from build123d import *

# Parameters (mm, degrees)
PAD_DEPTH       = 1.7
SKETCH002_W     = 6
SKETCH002_H     = 6
PAD009_DEPTH    = 4.52
SKETCH022_W     = 5
SKETCH022_H     = 3.52
SKETCH022_W_2   = 0.5
SKETCH022_H_2   = 0.5
POCKET011_DEPTH = 5
SKETCH023_W     = 0.5
SKETCH023_H     = 1.6
SKETCH023_W_2   = 1.6
SKETCH023_H_2   = 0.5
POCKET012_DEPTH = 2
FILLET015_R     = 0.2


with BuildPart() as part:
    # Sketch → Pad (new body)
    with BuildSketch(Plane.XY):
        with BuildLine():
            Line((0, 0), (30, 0))
            Line((30, 0), (30, 1))
            Line((30, 1), (31, 1))
            Line((31, 1), (31, 18.27))
            Line((31, 18.27), (24.4, 18.27))
            ThreePointArc((24.4, 24.87), (21.1, 21.57), (24.4, 18.27))
            Line((24.4, 24.87), (31, 24.87))
            Line((31, 24.87), (31, 59.13))
            Line((31, 59.13), (24.4, 59.13))
            ThreePointArc((24.4, 65.73), (21.1, 62.43), (24.4, 59.13))
            Line((24.4, 65.73), (31, 65.73))
            Line((31, 65.73), (31, 83))
            Line((30, 83), (31, 83))
            Line((30, 84), (30, 83))
            Line((30, 84), (0, 84))
            Line((0, 84), (-30, 84))
            Line((-30, 84), (-30, 83))
            Line((-30, 83), (-31, 83))
            Line((-31, 83), (-31, 65.73))
            Line((-31, 65.73), (-24.4, 65.73))
            ThreePointArc((-24.4, 59.13), (-21.1, 62.43), (-24.4, 65.73))
            Line((-24.4, 59.13), (-31, 59.13))
            Line((-31, 59.13), (-31, 24.87))
            Line((-31, 24.87), (-24.4, 24.87))
            ThreePointArc((-24.4, 18.27), (-21.1, 21.57), (-24.4, 24.87))
            Line((-24.4, 18.27), (-31, 18.27))
            Line((-31, 18.27), (-31, 1))
            Line((-31, 1), (-30, 1))
            Line((-30, 1), (-30, 0))
            Line((-30, 0), (0, 0))
        make_face()
    extrude(amount=PAD_DEPTH)

    # Sketch002 → Pad009 (new body)
    with BuildSketch(Plane.XY.offset(1.7)):
        with Locations((-12.43, 85.03)):
            Rectangle(SKETCH002_W, SKETCH002_H)
    extrude(amount=PAD009_DEPTH)

    # Sketch022 → Pocket011 (cut)
    with BuildSketch(Plane(origin=(0, 88.03, 0), x_dir=(-1, 0, 0), z_dir=(0, 1, 0))):
        with Locations((12.43, 3.96)):
            Rectangle(SKETCH022_W, SKETCH022_H)
        with Locations((11.5, 4.51)):
            Rectangle(SKETCH022_W_2, SKETCH022_H_2, mode=Mode.SUBTRACT)
        with Locations((13.5, 4.51)):
            Rectangle(SKETCH022_W_2, SKETCH022_H_2, mode=Mode.SUBTRACT)
    extrude(amount=-POCKET011_DEPTH, mode=Mode.SUBTRACT)

    # Sketch023 → Pocket012 (cut)
    with BuildSketch(Plane(origin=(0, 88.03, 0), x_dir=(-1, 0, 0), z_dir=(0, 1, 0))):
        with Locations((9.68, 4.02)):
            Rectangle(SKETCH023_W, SKETCH023_H)
        with Locations((15.18, 4.02)):
            Rectangle(SKETCH023_W, SKETCH023_H)
        with Locations((12.45003, 5.97)):
            Rectangle(SKETCH023_W_2, SKETCH023_H_2)
    extrude(amount=-POCKET012_DEPTH, mode=Mode.SUBTRACT)

    # Fillet015
    fillet015_edges = [part.edges().sort_by_distance(p)[0] for p in [
        (-13.5, 88.03, 4.76),
        (-13.75, 88.03, 4.51),
        (-13.5, 88.03, 4.26),
        (-13.25, 88.03, 4.51),
        (-11.5, 88.03, 4.76),
        (-11.75, 88.03, 4.51),
        (-11.5, 88.03, 4.26),
        (-11.25, 88.03, 4.51),
    ]]
    fillet(fillet015_edges, radius=FILLET015_R)


solid = part.part
Geometry: final body of the model. Coordinates: model frame, mm. A direction names the side the tool comes from. Coordinates: 2 decimals unless noted, no trailing zeros. Order: outer loops, then holes, each group sorted by start corner. A loop starts at its lowest first (then second) coordinate and runs counter-clockwise, first axis right, second up.
(1) First-contact query: pin 1 (3.5 mm diameter, centred on y = 86, z = 3.5, fed in from +X); pin 2 (0.5 mm diameter, centred on x = 26, z = 1.5, fed in from +Y); pin 3 (2 mm diameter, centred on y = 57, z = 3, fed in from +X); pin 4 (0.5 mm diameter, centred on x = 30.5, z = 0.5, fed in from -Y). Flat tips, straight axial feed; report the tip coordinate or a pass-through.
(2) Draft query along X for faces 1 (the face through (-28, 59.13, 1)), 2 (the face through (-12.4, 85.6, 5.72)), 3 (the face through (31, 42, 1)). Return one class per face: pulls with the +X half, pulls with the -X half, needs draft (parallel to the pull), parting line crosses it, or undercut.
(3) Section query A-A (y = 62.43). Return the cut outline in (x, z).
(4) Material intervals for probe 1 along Y at (x, z) = (-27, 1.5); probe 2 along Z at (x, y) = (18.5, 41); probe 3 along Y at (x, z) = (-11, 4.5), sorted ascending.
(5) Section query B-B (x = 2). Return the cut outline in (y, z), plus the area to 3 significant figures.
(6) Access query for faces 4 (the face through (28, 59.13, 1)), 5 (the face through (-12, 86, 1.7)), 6 (the face through (-9.43, 85, 4)), 7 (the face through (-28, 65.73, 1)), 8 (the face through (-9.93, 85, 4)). Directions: +Z, -Z, +X, -X, +Y, -Y. A direction counts if a zero-diameter tool reaches every point of the face in a straight line with its end or side. Return the directions, or none.
Solution:
1. pin 1: stops at x = -9.43
1. pin 2: stops at y = 84
1. pin 3: passes through
1. pin 4: stops at y = 1
2. face 1: needs draft
2. face 2: undercut
2. face 3: pulls with the +X half
3. outline: (-21.1, 0) - (21.1, 0) - (21.1, 1.7) - (-21.1, 1.7) - close
4. probe 1: y = 0 to 18.27, 24.87 to 59.13, 65.73 to 84
4. probe 2: z = 0 to 1.7
4. probe 3: y = 82.03 to 83.03
5. outline: (0, 0) - (84, 0) - (84, 1.7) - (0, 1.7) - close
5. area: 143 mm2
6. face 4: +Z, -Z, +X
6. face 5: -Z, +X, -X, +Y
6. face 6: +Z, +X, +Y, -Y
6. face 7: +Z, -Z, -X
6. face 8: +Y
